For this review, use the dimensioned drawing (mm, ordinates from the lowest corner) and the shaded views. Give positions to 0.01 mm unless a question says otherwise; leave off trailing zeros. Order: outer loops, then holes, each group sorted by start corner. A loop starts at its lowest first (then second) coordinate and runs counter-clockwise, first axis right, second up. Notation, with made-up numbers: (23, 28) - (45, 28) arc R20 cw to (45, 39) - close; hole circle Ø3 at (6.5, -31). An arc over 180 degrees is marked (long way). One line per item, written item: value.
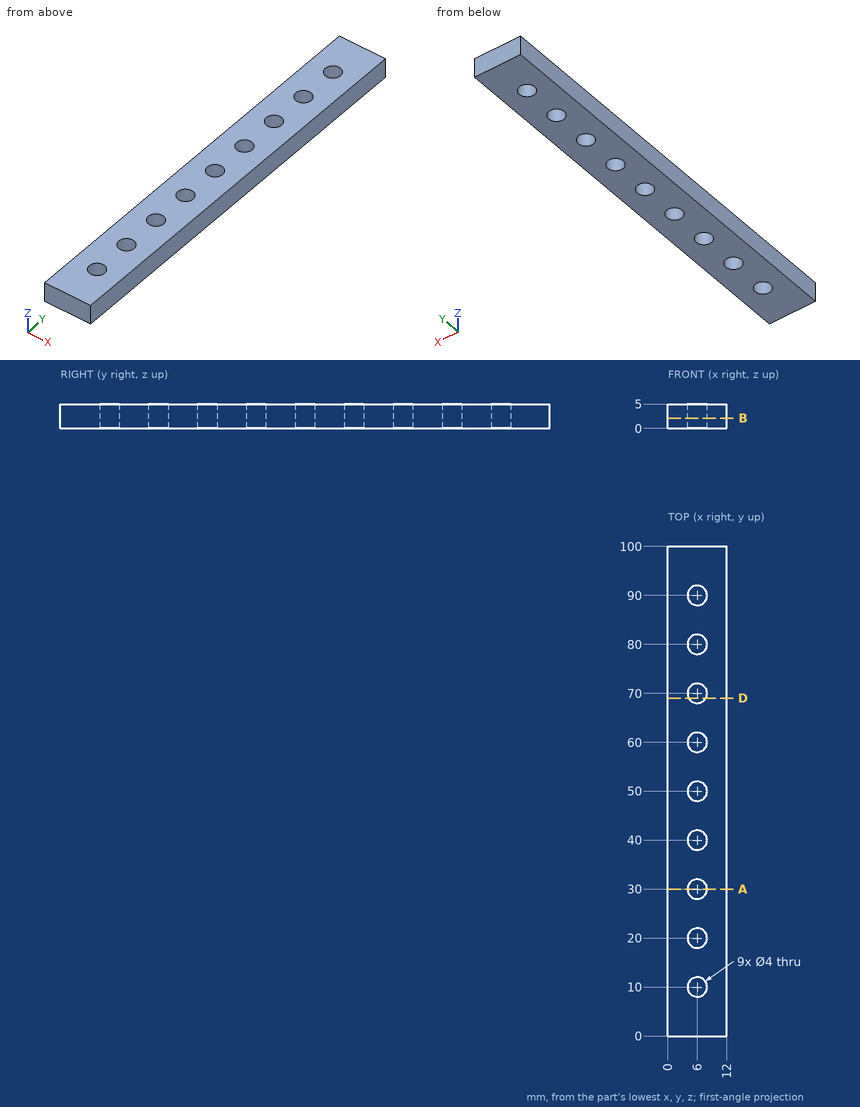
(1) For P1, Ø3, axis at x = 6, y = 50, coming from the +Z side, flat-tipped, find the tip position at first contact; note if it passes through.
Answers below:
P1: passes through
(2) Take a section at D-D (y = 69). Write out the cut boundary in (x, z), then the cut area to 3 significant figures.
Answers below:
outline: (0, 0) - (4.27, 0) - (4.27, 5) - (0, 5) - close; (7.73, 0) - (12, 0) - (12, 5) - (7.73, 5) - close
area: 42.7 mm^2
(3) Take a section at B-B (z = 2.1). Give the number of separate pieces and of enclosed holes in the cut face, then the cut area to 3 significant figures.
Answers below:
separate pieces: 1
enclosed holes: 9
area: 1,090 mm^2
(4) Wall thickness on line 1 (X direction, y = 70, z = 3.85): over which ranges is the line inside the solid? List them lowest first. Write a range as from..to.
Answers below:
line 1: x = 0..4, 8..12
(5) Take a section at A-A (y = 30). Write out the cut boundary in (x, z).
Answers below:
outline: (0, 0) - (4, 0) - (4, 5) - (0, 5) - close; (8, 0) - (12, 0) - (12, 5) - (8, 5) - close
